```python
from build123d import *

# Parameters (mm, degrees)
SKETCH1_R           = 11
BOSS_EXTRUDE1_DEPTH = 7
SKETCH2_W           = 5
SKETCH2_H           = 2.5
BOSS_EXTRUDE2_DEPTH = 13
CHAMFER2_SIZE       = 2
BOSS_EXTRUDE6_DEPTH = 2.5
CHAMFER3_SIZE       = 2
CHAMFER4_SIZE       = 2
BOSS_EXTRUDE4_DEPTH = 2.5
CHAMFER6_SIZE       = 2.5
CHAMFER7_SIZE       = 7
CHAMFER7_SIZE_2     = 13.165085257
CUT_EXTRUDE1_START  = -3
SKETCH6_R           = 2
CUT_EXTRUDE1_DEPTH  = 2.5
SKETCH7_R           = 2
CUT_EXTRUDE2_DEPTH  = 6


with BuildPart() as part:
    # Sketch1 → Boss-Extrude1 (new body)
    with BuildSketch(Plane.XY):
        Polygon((-15, 11.5), (-12.5, 14), (12.5, 14), (15, 11.5), (15, -14), (-15, -14), align=None)
        Circle(SKETCH1_R, mode=Mode.SUBTRACT)
    extrude(amount=BOSS_EXTRUDE1_DEPTH)

    # Sketch2 → Boss-Extrude2 (add)
    with BuildSketch(Plane(origin=(0, 0, 0), x_dir=(-1, 0, 0), z_dir=(0, 0, -1))):
        with Locations((-12.5, -12.75)):
            Rectangle(SKETCH2_W, SKETCH2_H)
        with Locations((12.5, -12.75)):
            Rectangle(SKETCH2_W, SKETCH2_H)
    extrude(amount=BOSS_EXTRUDE2_DEPTH)

    # Chamfer2
    chamfer2_edges = [part.edges().sort_by_distance(p)[0] for p in [
        (-10, -12.75, 0),
        (10, -12.75, 0),
    ]]
    chamfer(chamfer2_edges, length=CHAMFER2_SIZE)

    # Sketch5 → Boss-Extrude6 (add)
    with BuildSketch(Plane.XZ.offset(14)):
        Polygon((-10, -2), (-10, -7.5), (10, -7.5), (10, -2), (8, 0), (-8, 0), align=None)
    extrude(amount=-BOSS_EXTRUDE6_DEPTH)

    # Chamfer3
    chamfer3_edges = [part.edges().sort_by_distance(p)[0] for p in [
        (15, -1.25, 7),
    ]]
    chamfer(chamfer3_edges, length=CHAMFER3_SIZE)

    # Chamfer4
    chamfer4_edges = [part.edges().sort_by_distance(p)[0] for p in [
        (-15, -1.25, 7),
    ]]
    chamfer(chamfer4_edges, length=CHAMFER4_SIZE)

    # Sketch4 → Boss-Extrude4 (add)
    with BuildSketch(Plane(origin=(0, 0, 0), x_dir=(-1, 0, 0), z_dir=(0, 0, -1))):
        Polygon((-15, -1.25), (15, 11.5), (12.5, 14), (-12.5, 14), (-15, 11.5), align=None)
    extrude(amount=BOSS_EXTRUDE4_DEPTH)

    # Chamfer6
    # the kernel refuses this chamfer: 2.5 mm, written as the material it adds along each edge
    with BuildSketch(Plane(origin=(20.916998416, -3.764724327, 0), x_dir=(-0.39099275668343275, -0.9199829569021947, 0.02749587661058635), z_dir=(-0.9203309184584746, 0.39114064034485174, 0))) as chamfer6_piece_1_section:
        Polygon((CHAMFER6_SIZE * 0.999621916911, -CHAMFER6_SIZE * 0.0274958766106), (-CHAMFER6_SIZE * 0.0274958766106, -CHAMFER6_SIZE * 0.999621916911), (0, 0), align=None)
    chamfer6_piece_1 = extrude(amount=17.214861222, mode=Mode.PRIVATE)
    chamfer6_piece_1 = chamfer6_piece_1 - Plane(origin=(0, 0, -0.830769879), x_dir=(1, 0, 0), z_dir=(0, 0, -1)) * Cylinder(11, 45, mode=Mode.PRIVATE)
    chamfer6_piece_1 = split(chamfer6_piece_1, bisect_by=Plane(origin=(15, -1.305255327, -0.830769879), z_dir=(-1, 0, 0)), keep=Keep.TOP, mode=Mode.PRIVATE)
    add(chamfer6_piece_1)
    with BuildSketch(Plane(origin=(-1.383846422, 5.71313473, 0), x_dir=(-0.39099275668343275, -0.9199829569021946, 0.02749587661058637), z_dir=(-0.9203309184584746, 0.39114064034485174, 0))) as chamfer6_piece_2_section:
        Polygon((CHAMFER6_SIZE * 0.999621916911, -CHAMFER6_SIZE * 0.0274958766106), (-CHAMFER6_SIZE * 0.0274958766106, -CHAMFER6_SIZE * 0.999621916911), (0, 0), align=None)
    chamfer6_piece_2 = extrude(amount=21.224052785, mode=Mode.PRIVATE)
    chamfer6_piece_2 = chamfer6_piece_2 - Plane(origin=(0, 0, -0.851096237), x_dir=(1, 0, 0), z_dir=(0, 0, -1)) * Cylinder(11, 53, mode=Mode.PRIVATE)
    chamfer6_piece_2 = split(chamfer6_piece_2, bisect_by=Plane(origin=(-15, 9.126408424, -0.851096237), z_dir=(1, 0, 0)), keep=Keep.TOP, mode=Mode.PRIVATE)
    add(chamfer6_piece_2)

    # Chamfer7
    # the kernel refuses this chamfer: 13.165085257, 7 mm, written as the material it adds along each edge
    with BuildSketch(Plane(origin=(-15, -11.5, 0), x_dir=(0, 0.9979482451756082, 0.06402577567608186), z_dir=(1, 0, 0))) as chamfer7_piece_1_section:
        Polygon((CHAMFER7_SIZE * 0.997948245176, -CHAMFER7_SIZE * 0.0640257756761), (-CHAMFER7_SIZE_2 * 0.0640257756781, -CHAMFER7_SIZE_2 * 0.997948245208), (0, 0), align=None)
    chamfer7_piece_1 = extrude(amount=30, mode=Mode.PRIVATE)
    chamfer7_piece_1 = chamfer7_piece_1 - Plane(origin=(0, 0, -3.073682767), x_dir=(1, 0, 0), z_dir=(0, 0, -1)) * Cylinder(11, 113, mode=Mode.PRIVATE)
    chamfer7_piece_1 = split(chamfer7_piece_1, bisect_by=Plane(origin=(-12.500128058, -8.887755394, -7.5), z_dir=(0, 0, 1)), keep=Keep.TOP, mode=Mode.PRIVATE)
    chamfer7_piece_1 = split(chamfer7_piece_1, bisect_by=Plane(origin=(-10, -8.887755394, -3.073682767), z_dir=(-1, 0, 0)), keep=Keep.TOP, mode=Mode.PRIVATE)
    add(chamfer7_piece_1)
    with BuildSketch(Plane(origin=(-15, -11.5, 0), x_dir=(0, 0.9979482451756082, 0.06402577567608186), z_dir=(1, 0, 0))) as chamfer7_piece_2_section:
        Polygon((CHAMFER7_SIZE * 0.997948245176, -CHAMFER7_SIZE * 0.0640257756761), (-CHAMFER7_SIZE_2 * 0.0640257756781, -CHAMFER7_SIZE_2 * 0.997948245208), (0, 0), align=None)
    chamfer7_piece_2 = extrude(amount=30, mode=Mode.PRIVATE)
    chamfer7_piece_2 = split(chamfer7_piece_2, bisect_by=Plane(origin=(-12.5, -10.721530873, -7.5), z_dir=(0, 0, -1)), keep=Keep.TOP, mode=Mode.PRIVATE)
    chamfer7_piece_2 = split(chamfer7_piece_2, bisect_by=Plane(origin=(-10, -10.721530873, -9.597564575), z_dir=(-1, 0, 0)), keep=Keep.TOP, mode=Mode.PRIVATE)
    chamfer7_piece_2 = split(chamfer7_piece_2, bisect_by=Plane(origin=(-12.5, -10.721530873, -13), z_dir=(0, 0, 1)), keep=Keep.TOP, mode=Mode.PRIVATE)
    add(chamfer7_piece_2)
    with BuildSketch(Plane(origin=(-15, -11.5, 0), x_dir=(0, 0.9979482451756082, 0.06402577567608186), z_dir=(1, 0, 0))) as chamfer7_piece_3_section:
        Polygon((CHAMFER7_SIZE * 0.997948245176, -CHAMFER7_SIZE * 0.0640257756761), (-CHAMFER7_SIZE_2 * 0.0640257756781, -CHAMFER7_SIZE_2 * 0.997948245208), (0, 0), align=None)
    chamfer7_piece_3 = extrude(amount=30, mode=Mode.PRIVATE)
    chamfer7_piece_3 = chamfer7_piece_3 - Plane(origin=(0, 0, -3.793876077), x_dir=(1, 0, 0), z_dir=(0, 0, -1)) * Cylinder(11, 113, mode=Mode.PRIVATE)
    chamfer7_piece_3 = split(chamfer7_piece_3, bisect_by=Plane(origin=(-9.499486782, -6.598719884, -7.5), z_dir=(0, 0, 1)), keep=Keep.TOP, mode=Mode.PRIVATE)
    chamfer7_piece_3 = split(chamfer7_piece_3, bisect_by=Plane(origin=(10, -6.598719884, -3.793876077), z_dir=(-1, 0, 0)), keep=Keep.TOP, mode=Mode.PRIVATE)
    chamfer7_piece_3 = split(chamfer7_piece_3, bisect_by=Plane(origin=(-10, -6.598719884, -3.793876077), z_dir=(1, 0, 0)), keep=Keep.TOP, mode=Mode.PRIVATE)
    add(chamfer7_piece_3)
    with BuildSketch(Plane(origin=(-15, -11.5, 0), x_dir=(0, 0.9979482451756082, 0.06402577567608186), z_dir=(1, 0, 0))) as chamfer7_piece_4_section:
        Polygon((CHAMFER7_SIZE * 0.997948245176, -CHAMFER7_SIZE * 0.0640257756761), (-CHAMFER7_SIZE_2 * 0.0640257756781, -CHAMFER7_SIZE_2 * 0.997948245208), (0, 0), align=None)
    chamfer7_piece_4 = extrude(amount=30, mode=Mode.PRIVATE)
    chamfer7_piece_4 = split(chamfer7_piece_4, bisect_by=Plane(origin=(12.5, -10.721530873, -7.5), z_dir=(0, 0, -1)), keep=Keep.TOP, mode=Mode.PRIVATE)
    chamfer7_piece_4 = split(chamfer7_piece_4, bisect_by=Plane(origin=(10, -10.721530873, -9.597564575), z_dir=(1, 0, 0)), keep=Keep.TOP, mode=Mode.PRIVATE)
    chamfer7_piece_4 = split(chamfer7_piece_4, bisect_by=Plane(origin=(12.5, -10.721530873, -13), z_dir=(0, 0, 1)), keep=Keep.TOP, mode=Mode.PRIVATE)
    add(chamfer7_piece_4)
    with BuildSketch(Plane(origin=(-15, -11.5, 0), x_dir=(0, 0.9979482451756082, 0.06402577567608186), z_dir=(1, 0, 0))) as chamfer7_piece_5_section:
        Polygon((CHAMFER7_SIZE * 0.997948245176, -CHAMFER7_SIZE * 0.0640257756761), (-CHAMFER7_SIZE_2 * 0.0640257756781, -CHAMFER7_SIZE_2 * 0.997948245208), (0, 0), align=None)
    chamfer7_piece_5 = extrude(amount=30, mode=Mode.PRIVATE)
    chamfer7_piece_5 = chamfer7_piece_5 - Plane(origin=(0, 0, -3.073682766), x_dir=(1, 0, 0), z_dir=(0, 0, -1)) * Cylinder(11, 113, mode=Mode.PRIVATE)
    chamfer7_piece_5 = split(chamfer7_piece_5, bisect_by=Plane(origin=(12.500128057, -8.887755394, -7.5), z_dir=(0, 0, 1)), keep=Keep.TOP, mode=Mode.PRIVATE)
    chamfer7_piece_5 = split(chamfer7_piece_5, bisect_by=Plane(origin=(10, -8.887755394, -3.073682766), z_dir=(1, 0, 0)), keep=Keep.TOP, mode=Mode.PRIVATE)
    add(chamfer7_piece_5)

    # Sketch6 → Cut-Extrude1 (cut)
    # profile 1 of 2: a face of its own
    with BuildSketch(Plane.XZ.offset(14).offset(CUT_EXTRUDE1_START)):
        Polygon((-7.55, 0.508141571), (-7.55, 4.491858429), (-11, 6.483716857), (-14.45, 4.491858429), (-14.45, 0.508141571), (-11, -1.483716857), align=None)
        with Locations(Location((-11, 2.5, 0), (0, 0, 270))):
            Circle(SKETCH6_R, mode=Mode.SUBTRACT)
    # profile 2 of 2: a face of its own
    with BuildSketch(Plane.XZ.offset(14).offset(CUT_EXTRUDE1_START)):
        Polygon((11, -1.483716857), (7.55, 0.508141571), (7.55, 4.491858429), (11, 6.483716857), (14.45, 4.491858429), (14.45, 0.508141571), align=None)
    extrude(amount=-CUT_EXTRUDE1_DEPTH, mode=Mode.SUBTRACT)

    # Sketch7 → Cut-Extrude2 (cut)
    with BuildSketch(Plane.XZ.offset(14)):
        with Locations(Location((11, 2.5, 0), (0, 0, 270))):
            Circle(SKETCH7_R)
        with Locations(Location((-11, 2.5, 0), (0, 0, 270))):
            Circle(SKETCH7_R)
    extrude(amount=-CUT_EXTRUDE2_DEPTH, mode=Mode.SUBTRACT)


solid = part.part
```
Could you check a few things on this model? Use its own coordinates, in mm. A direction names the side the tool comes from. Coordinates: 2 decimals unless noted, no trailing zeros. Write each loop counter-clockwise with the first axis right and the second up, starting at its lowest first coordinate (ties: lowest second). Pieces come first, ordered by that corner, then holes. Notation, with made-up numbers: M 12,54 L 60,54 A10 cw 60,58 Z; hole C 89.25,45 d5. An arc over 180 degrees is marked long. Answer as CSV lines item,"result". Start each with the question number.
1) I want a section at B-B, the plane x = -6.5. Please give me the cut outline in (y, z), and give its area (3 significant figures).
2) For faces 5 (the flat face through (9.3, -9.8, -0.5)), 6 (the cylindrical face through (-2.017, -10.813, 1.26)), 7 (the cylindrical face through (12.983, -12.521, 2.76)), which set-ups out of +Z, -Z, +X, -X, +Y, -Y let a thin tool reach every point of the face, with its end or its side?
3) I want a section at C-C, the plane y = -0.75. Please give me the cut outline in (x, z).
4) Please list where these lines run through material, in increasing order: line 1 (X direction, y = -12.25, z = 2.5); line 2 (Y direction, x = 13.5, z = 1.5); line 3 (Y direction, x = -8, z = 5). Write a range as from..to.
5) We'd pull the mould along Z, two halves only. Please class faces 1 (the flat face through (-13, -13, -13)), 2 (the flat face through (2, 7, 0)), 3 (the flat face through (0, 14, 2)), 4 (the flat face through (14.45, -10, 3)): +Z half, -Z half, draft (parallel to the pull), parting line (faces both ways), or undercut.
6) I want a section at D-D, the plane z = -9. Please give me the cut outline in (x, y), and give its area (3 significant figures).
7) For P1, Ø6, axis at x = -2.5, y = 7, coming from the +Z side; P2, Ø3, axis at x = -11, z = 2.5, coming from the -Y side; P3, Ø8, axis at x = -10, y = 5, coming from the -Z side, each with a flat end and sliding along its axis, tell me the tip position at first contact or that it passes through.
Data:
1,outline,"M -14,-7.5 L -8.87,-7.5 L -8.87,7 L -14,7 Z; M 7.89,-2.5 L 14,-2.5 L 14,7 L 8.87,7 L 8.87,0 L 7.89,0 Z"
1,area,"125 mm^2"
2,face 5,"none"
2,face 6,"+Z"
2,face 7,"-Y"
3,outline,"M -15,0 L -10.97,0 L -10.97,7 L -13,7 L -15,5 Z; M 10.97,-1.39 L 13.82,-2.5 L 15,-2.5 L 15,5 L 13,7 L 10.97,7 Z"
4,line 1,"x = -15..-13, -9..9, 13..15"
4,line 2,"y = -14..-11, -8.5..13"
4,line 3,"y = -14..-7.55, 7.55..14"
5,face 1,"-Z half"
5,face 2,"+Z half"
5,face 3,"draft"
5,face 4,"undercut"
6,outline,"M -15,-14 L -10,-14 L -10,-9.29 L -15,-9.29 Z; M 10,-14 L 15,-14 L 15,-9.29 L 10,-9.29 Z"
6,area,"47.1 mm^2"
7,P1,"stops at z = 0"
7,P2,"stops at y = -8"
7,P3,"stops at z = -2.47"
